Design review of the part shown in the three views and the two pictorial views. Dimensions are in mm from the part's minimum x, y and z. A direction names the side the tool comes from. Give positions to 0.01 mm unless a question says otherwise; leave off trailing zeros. Write each loop counter-clockwise with the first axis right and the second up, starting at its lowest first coordinate (ties: lowest second). Pieces come first, ordered by that corner, then holes. Notation, with made-up numbers: (-38.5, 21) -> (-20.5, 21) arc R24 cw to (-20.5, 35) -> close; hole circle Ø2 at (67.5, 75.5). An arc over 180 degrees is marked (long way). Use CSV: the item, a comma, the result in double quotes.
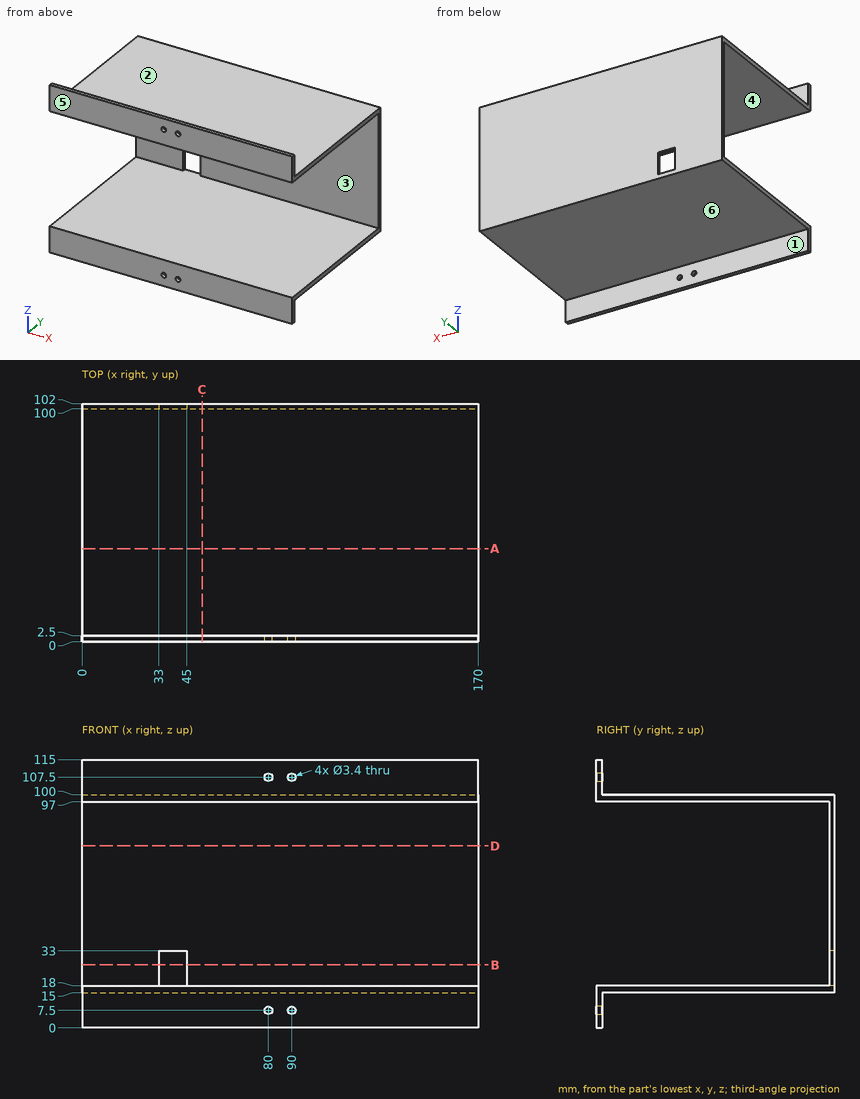
Q1. Insertion check: pin 1 (6 mm diameter, centred on x = 76.5, z = 51, fed in from -Y); pin 2 (3 mm diameter, centred on x = 66.5, y = 35, fed in from -Z); pin 3 (7.5 mm diameter, centred on x = 78, z = 107, fed in from +Y). Each pin has a flat end and moves straight along its axis. Give the tip position at first contact, or say it passes through.
Derived:
pin 1,"stops at y = 100"
pin 2,"stops at z = 15"
pin 3,"stops at y = 2.5"
Q2. Consider section C-C (x = 51.5). Write out the cut boundary in (y, z).
Derived:
outline,"(0, 0) -> (2.5, 0) -> (2.5, 15) -> (102, 15) -> (102, 100) -> (2.5, 100) -> (2.5, 115) -> (0, 115) -> (0, 97) -> (100, 97) -> (100, 18) -> (0, 18) -> close"
Q3. Consider section B-B (z = 27). Write out the cut boundary in (x, y).
Derived:
outline,"(0, 100) -> (33, 100) -> (33, 102) -> (0, 102) -> close; (45, 100) -> (170, 100) -> (170, 102) -> (45, 102) -> close"
Q4. The part is to be moulded in two halves that separate along Z. For the marked faces 4, 5 and 6, say which applies: pulls with the +Z half, pulls with the -Z half, needs draft (parallel to the pull), parting line crosses it, or undercut.
Derived:
face 4,"undercut"
face 5,"needs draft"
face 6,"pulls with the -Z half"
Q5. To check wall thickness, follow probe 1 along X at (y, z) = (1.75, 107.5); probe 2 along Z at (x, y) = (101.5, 98); probe 3 along Z at (x, y) = (80, 1.1). State the ranges of each line that lie inside material, in increasing order.
Derived:
probe 1,"x = 0 to 78.3, 81.7 to 88.3, 91.7 to 170"
probe 2,"z = 15 to 18, 97 to 100"
probe 3,"z = 0 to 5.8, 9.2 to 18, 97 to 105.8, 109.2 to 115"
Q6. Consider section D-D (z = 78). Write out the cut boundary in (x, y).
Derived:
outline,"(0, 100) -> (170, 100) -> (170, 102) -> (0, 102) -> close"
Q7. Machinability: for the marked faces 1, 2 and 3, which of the approach directions +Z, -Z, +X, -X, +Y, -Y give a long, thin tool a straight path to every point of the face, cutting with its end or side? Answer none if there is none.
Derived:
face 1,"-Z, +X, -X, +Y"
face 2,"+Z, +X, -X, +Y"
face 3,"+X, -X, -Y"
Q8. Consider section A-A (y = 40). Write out the cut boundary in (x, z).
Derived:
outline,"(0, 15) -> (170, 15) -> (170, 18) -> (0, 18) -> close; (0, 97) -> (170, 97) -> (170, 100) -> (0, 100) -> close"
